Could you check a few things on this model? Use its own coordinates, in mm. A direction names the side the tool comes from. Coordinates: 2 decimals unless noted, no trailing zeros. Write each loop counter-clockwise with the first axis right and the second up, starting at its lowest first coordinate (ties: lowest second). Pieces come first, ordered by that corner, then holes. Notation, with made-up numbers: (74, 69) - (85, 69) arc R12 ccw to (85, 74) - close; hole circle Ø11 at (-13.5, 19.25). An arc over 180 degrees is marked (long way). Answer as a JSON object with one key per item and string values. Group by question number.
1) Please list where these lines run through material, in increasing order: line 1 along X through (y, z) = (2.8, -0.5); line 2 along X through (y, z) = (0.25, 31); line 3 along Z through (x, y) = (-10, 1.95).
2) We'd pull the mould along X, two halves only. Please class faces 4 (the flat face through (-20, 1.48, 35.03)), 5 (the flat face through (-11.39, 1, -3)), 6 (the flat face through (11.39, 1, -3)), 7 (the flat face through (-5, 1, -6.1)): released by +X, released by -X, zero draft, split by the parting line, or undercut.
3) If we section it at A-A (z = 3): Write out the boundary of the cut face in (x, y).
4) If we section it at C-C (z = 17): Write out the boundary of the cut face in (x, y).
5) If we section it at B-B (x = 0): Write out the boundary of the cut face in (y, z), plus the area to 3 significant figures.
6) Will these pins go through, and if not, where does the flat tip stop? pin 1 Ø1 at (x, y) = (-22.5, 2.5) entering from -Z; pin 2 Ø1.5 at (y, z) = (1.5, 38) entering from +X; pin 3 Ø0.9 at (y, z) = (1, -2) entering from +X.
7) On a 3-axis mill with a long thin cutter (end or side, diameter ignored), from which of +Z, -Z, +X, -X, +Y, -Y can I reach the whole of each face in a straight line? I mean faces 1 (the flat face through (8.39, 1, 37)), 2 (the flat face through (-8.39, 1, -3)), 3 (the flat face through (20.79, 1.48, 0.17)). Say none if no direction works.
```python
from build123d import *

# Parameters (mm, degrees)
BOSS_EXTRUDE1_DEPTH = 3
FILLET1_R           = 4
FILLET2_R           = 1
FILLET3_R           = 7


with BuildPart() as part:
    # Sketch1 → Boss-Extrude1 (new body)
    with BuildSketch(Plane(origin=(0, 0, 0), x_dir=(1, 0, 0), z_dir=(0, 1, 0))):
        with BuildLine():
            Line((-1.5, 6.1), (-1.5, 0))
            ThreePointArc((-1.5, 0), (0, -1.5), (1.5, 0))
            Line((1.5, 0), (1.5, 6.1))
            Line((1.5, 6.1), (8.39, 6.1))
            Line((8.39, 6.1), (8.39, 0))
            ThreePointArc((8.39, 0), (9.89, -1.5), (11.39, 0))
            Line((11.39, 0), (11.39, 6.1))
            Line((11.39, 6.1), (21.345, 6.1))
            Line((21.345, 6.1), (20.121226415, -7.7))
            Line((20.121226415, -7.7), (26.121226415, -7.7))
            Line((26.121226415, -7.7), (27.123301887, 3.6))
            Line((27.123301887, 3.6), (30.353301887, 3.6))
            Line((30.353301887, 3.6), (27.375, -27.7))
            Line((27.375, -27.7), (19.725, -30.65))
            Line((19.725, -30.65), (20.405, -41.49))
            Line((20.405, -41.49), (17.97, -45.49))
            Line((17.97, -45.49), (11.39, -45.49))
            Line((11.39, -45.49), (11.39, -29.54))
            ThreePointArc((11.39, -29.54), (9.89, -28.04), (8.39, -29.54))
            Line((8.39, -29.54), (8.39, -45.49))
            Line((8.39, -45.49), (1.5, -45.49))
            Line((1.5, -45.49), (1.5, -29.54))
            ThreePointArc((1.5, -29.54), (0, -28.04), (-1.5, -29.54))
            Line((-1.5, -29.54), (-1.5, -45.49))
            Line((-1.5, -45.49), (-8.39, -45.49))
            Line((-8.39, -45.49), (-8.39, -29.54))
            ThreePointArc((-8.39, -29.54), (-9.89, -28.04), (-11.39, -29.54))
            Line((-11.39, -29.54), (-11.39, -45.49))
            Line((-11.39, -45.49), (-17.97, -45.49))
            Line((-17.97, -45.49), (-20.405, -41.49))
            Line((-20.405, -41.49), (-19.725, -30.65))
            Line((-19.725, -30.65), (-27.375, -27.7))
            Line((-27.375, -27.7), (-30.353301887, 3.6))
            Line((-30.353301887, 3.6), (-27.123301887, 3.6))
            Line((-27.123301887, 3.6), (-26.121226415, -7.7))
            Line((-26.121226415, -7.7), (-20.121226415, -7.7))
            Line((-20.121226415, -7.7), (-21.345, 6.1))
            Line((-21.345, 6.1), (-11.39, 6.1))
            Line((-11.39, 6.1), (-11.39, 0))
            ThreePointArc((-11.39, 0), (-9.89, -1.5), (-8.39, 0))
            Line((-8.39, 0), (-8.39, 6.1))
            Line((-8.39, 6.1), (-1.5, 6.1))
        make_face()
    extrude(amount=BOSS_EXTRUDE1_DEPTH)

    # Fillet1
    # the kernel refuses this fillet: 4 mm, written as the material it takes off along each edge
    with BuildSketch(Plane(origin=(-30.353301887, -10.570685878, -3.6), x_dir=(0.09472555048973348, 0, 0.9955034254508706), z_dir=(0, 1, 0))) as fillet1_piece_1:
        with BuildLine():
            CenterArc((4.228274351, 4), FILLET1_R, 191.310800098, 78.689199902)
            Line((0.305963528, 3.215476064), (0.227517312, 3.199785585))
            ThreePointArc((0.227517312, 3.199785585), (0.07334149, 1.615316076), (-0.079640274, 0.007578044))
            Line((-0.079640274, 0.007578044), (0, -0.08))
            Line((0, -0.08), (4.228274351, -0.08))
            Line((4.228274351, -0.08), (4.228274351, 0))
        make_face()
    extrude(amount=24.141371757, mode=Mode.SUBTRACT)
    with BuildSketch(Plane(origin=(30.353301887, -10.570685878, -3.6), x_dir=(-1, 0, 0), z_dir=(0, 1, 0))) as fillet1_piece_2:
        with BuildLine():
            CenterArc((4.382539317, 3.830359399), FILLET1_R, 174.564476221, 78.689199902)
            Line((0.400525616, 4.2092616), (0.320885342, 4.216839645))
            Line((0.320885342, 4.216839645), (-0.079640274, 0.007578044))
            Line((-0.079640274, 0.007578044), (0, -0.08))
            ThreePointArc((0, -0.08), (1.615, -0.08), (3.206949214, -0.076607188))
            Line((3.206949214, -0.076607188), (3.23, 0))
        make_face()
    extrude(amount=24.141371757, mode=Mode.SUBTRACT)

    # Fillet2
    fillet2_edges = [part.edges().sort_by_distance(p)[0] for p in [
        (20.121226415, 1.5, 7.7),
        (26.121226415, 1.5, 7.7),
        (-26.121226415, 1.5, 7.7),
        (-20.121226415, 1.5, 7.7),
    ]]
    fillet(fillet2_edges, radius=FILLET2_R)

    # Fillet3
    # the kernel refuses this fillet: 7 mm, written as the material it takes off along each edge
    with BuildSketch(Plane(origin=(-17.97, -9.834409558, 45.49), x_dir=(-0.5199808190603072, 0, -0.8541779368547118), z_dir=(0, 1, 0)), Plane(origin=(17.97, -9.834409558, 45.49), x_dir=(-1, 0, 0), z_dir=(0, 1, 0))) as fillet3_piece_1:
        with BuildLine():
            CenterArc((FILLET3_R * 0.561966260458, -FILLET3_R), FILLET3_R, 90, 58.669035113)
            Line((-FILLET3_R * 0.292211676397, -FILLET3_R * 0.48001918094), (0, 0))
            Line((0, 0), (FILLET3_R * 0.561966260458, 0))
        make_face()
    extrude(amount=22.668819116, mode=Mode.SUBTRACT)
    with BuildSketch(Plane(origin=(-20.405, -5.504377364, 41.49), x_dir=(0.0626075637538876, 0, -0.9980382221943221), z_dir=(0, 1, 0)), Plane(origin=(20.405, -5.504377364, 41.49), x_dir=(-0.5199808190603077, 0, 0.8541779368547114), z_dir=(0, 1, 0))) as fillet3_piece_2:
        with BuildLine():
            CenterArc((FILLET3_R * 0.314535849376, -FILLET3_R), FILLET3_R, 90, 34.920461628)
            Line((-FILLET3_R * 0.257902882493, -FILLET3_R * 0.180052502744), (0, 0))
            Line((0, 0), (FILLET3_R * 0.314535849376, 0))
        make_face()
    extrude(amount=14.008754728, mode=Mode.SUBTRACT)
    with BuildSketch(Plane(origin=(-27.375, -10.824428121, 27.7), x_dir=(-0.09472555048973366, 0, -0.9955034254508704), z_dir=(0, 1, 0)), Plane(origin=(27.375, -10.824428121, 27.7), x_dir=(-0.9330309060396333, 0, 0.3597962317407744), z_dir=(0, 1, 0))) as fillet3_piece_3:
        with BuildLine():
            CenterArc((FILLET3_R * 0.61853874979, -FILLET3_R), FILLET3_R, 90, 63.476793772)
            Line((-FILLET3_R * 0.276214817108, -FILLET3_R * 0.553439752639), (0, 0))
            Line((0, 0), (FILLET3_R * 0.61853874979, 0))
        make_face()
    extrude(amount=24.648856243, mode=Mode.SUBTRACT)


solid = part.part
```
Here are the results:
{
 "1": {"line 1": "x = -29.9 to -26.85, -20.85 to -11.39, -8.39 to -1.5, 1.5 to 8.39, 11.39 to 20.85, 26.85 to 29.9", "line 2": "x = -19.75 to -11.39, -8.39 to -1.5, 1.5 to 8.39, 11.39 to 19.75", "line 3": "z = 1.5 to 28.04"},
 "2": {"face 4": "released by -X", "face 5": "undercut", "face 6": "undercut", "face 7": "zero draft"},
 "3": {"outline": "(-29.73, 0) - (-26.54, 0) - (-26.54, 3) - (-29.73, 3) - close; (-20.54, 0) - (20.54, 0) - (20.54, 3) - (-20.54, 3) - close; (26.54, 0) - (29.73, 0) - (29.73, 3) - (26.54, 3) - close"},
 "4": {"outline": "(-28.39, 0) - (28.39, 0) - (28.39, 3) - (-28.39, 3) - close"},
 "5": {"outline": "(0, 1.5) - (3, 1.5) - (3, 28.04) - (0, 28.04) - close", "area": "79.6 mm²"},
 "6": {"pin 1": "stops at z = 7.7", "pin 2": "stops at x = 20.23", "pin 3": "stops at x = 29.55"},
 "7": {"face 1": "+Z, +Y, -Y", "face 2": "-Z, +Y, -Y", "face 3": "+Y, -Y"}
}
